Build history of the part. All positions in model axes, mm. Coordinates: 2 decimals unless noted, no trailing zeros. Write each loop counter-clockwise with the first axis right and the second up, starting at its lowest first coordinate (ties: lowest second). Pieces come first, ordered by that corner, then holes.
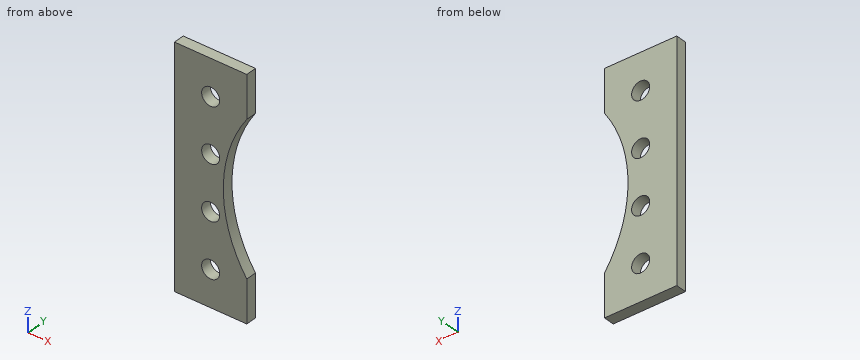
```python
from build123d import *

# Parameters (mm, degrees)
F0_R     = 5
F1_DEPTH = 6


# Not quite as in the source:
# - a feature names something its author has since deleted; it is built from what else it names


with BuildPart() as f1:
    # F0 (on Front) → F1 (new body)
    with BuildSketch(Plane.XZ):
        with BuildLine():
            Line((0, 130), (0, 0))
            Line((0, 0), (40, 0))
            Line((40, 0), (40, 23.4187542274))
            ThreePointArc((40, 23.4187542274), (27, 65), (40, 106.5812457726))
            Line((40, 106.5812457726), (40, 130))
            Line((40, 130), (35, 130))
            Line((35, 130), (0, 130))
        make_face()
        with Locations((20, 20)):
            Circle(F0_R, mode=Mode.SUBTRACT)
        with Locations((20, 50)):
            Circle(F0_R, mode=Mode.SUBTRACT)
        with Locations((20, 80)):
            Circle(F0_R, mode=Mode.SUBTRACT)
        with Locations((20, 110)):
            Circle(F0_R, mode=Mode.SUBTRACT)
    extrude(amount=F1_DEPTH)


solid = f1.part
```
1. Saw through at D-D on x = 29.5. List the corners of the cut face in (y, z), plus the area to 3 significant figures.
Computed values:
outline: (-6, 0) - (0, 0) - (0, 46.06) - (-6, 46.06) - close; (-6, 83.94) - (0, 83.94) - (0, 130) - (-6, 130) - close
area: 553 mm2
2. Saw through at C-C on y = -2.8. List the corners of the cut face in (x, z), plus the area to 3 significant figures.
Computed values:
outline: (0, 0) - (40, 0) - (40, 23.42) arc R73 cw to (40, 106.58) - (40, 130) - (0, 130) - close; hole circle Ø10 at (20, 20); hole circle Ø10 at (20, 50); hole circle Ø10 at (20, 80); hole circle Ø10 at (20, 110)
area: 4,150 mm2
3. Saw through at B-B on x = 20. List the corners of the cut face in (y, z), plus the area to 3 significant figures.
Computed values:
outline: (-6, 0) - (0, 0) - (0, 15) - (-6, 15) - close; (-6, 25) - (0, 25) - (0, 45) - (-6, 45) - close; (-6, 55) - (0, 55) - (0, 75) - (-6, 75) - close; (-6, 85) - (0, 85) - (0, 105) - (-6, 105) - close; (-6, 115) - (0, 115) - (0, 130) - (-6, 130) - close
area: 540 mm2
4. Saw through at A-A on z = 110. List the corners of the cut face in (x, y), plus the area to 3 significant figures.
Computed values:
outline: (0, -6) - (15, -6) - (15, 0) - (0, 0) - close; (25, -6) - (40, -6) - (40, 0) - (25, 0) - close
area: 180 mm2
5. Flat gauge pins, fed straight in: pin 1 (2 mm diameter, centred on y = -3.5, z = 59, fed in from +X); pin 2 (1.5 mm diameter, centred on y = -2, z = 49, fed in from +X). Where does each tip first touch, or does it go through?
Computed values:
pin 1: stops at x = 27.34
pin 2: stops at x = 28.95
6. Probe line 1 along Z through (x, y) = (20, -3.45); line 2 along Z through (x, y) = (21, -5.1); line 3 along Z through (x, y) = (34, -1.4). List the from-to ranges inside material, lowest first.
Computed values:
line 1: z = 0 to 15, 25 to 45, 55 to 75, 85 to 105, 115 to 130
line 2: z = 0 to 15.1, 24.9 to 45.1, 54.9 to 75.1, 84.9 to 105.1, 114.9 to 130
line 3: z = 0 to 33.81, 96.19 to 130
